```python
from build123d import *

# Parameters (mm, degrees)
SKETCH1_R           = 381
BOSS_EXTRUDE1_DEPTH = 12.7
SKETCH6_R           = 15.25
CUT_EXTRUDE1_DEPTH  = 12.7


with BuildPart() as part:
    # Sketch1 → Boss-Extrude1 (new body, symmetric)
    with BuildSketch(Plane(origin=(0, 0, 0), x_dir=(1, 0, 0), z_dir=(0, 1, 0))):
        Circle(SKETCH1_R)
    extrude(amount=BOSS_EXTRUDE1_DEPTH, both=True)

    # Sketch6 → Cut-Extrude1 (cut)
    with BuildSketch(Plane(origin=(0, 12.7, 0), x_dir=(1, 0, 0), z_dir=(0, 1, 0))):
        Circle(SKETCH6_R)
        with Locations((-101.6, 0)):
            Circle(SKETCH6_R)
        with Locations((101.6, 0)):
            Circle(SKETCH6_R)
        with Locations((-101.6, 101.6)):
            Circle(SKETCH6_R)
        with Locations((0, 101.6)):
            Circle(SKETCH6_R)
        with Locations((101.6, 101.6)):
            Circle(SKETCH6_R)
        with Locations((-101.6, -101.6)):
            Circle(SKETCH6_R)
        with Locations((0, -101.6)):
            Circle(SKETCH6_R)
        with Locations((101.6, -101.6)):
            Circle(SKETCH6_R)
        with Locations((101.6, 203.2)):
            Circle(SKETCH6_R)
        with Locations((0, 203.2)):
            Circle(SKETCH6_R)
        with Locations((-101.6, 203.2)):
            Circle(SKETCH6_R)
        with Locations((101.6, 304.8)):
            Circle(SKETCH6_R)
        with Locations((0, 304.8)):
            Circle(SKETCH6_R)
        with Locations((-101.6, 304.8)):
            Circle(SKETCH6_R)
        with Locations((101.6, -203.2)):
            Circle(SKETCH6_R)
        with Locations((0, -203.2)):
            Circle(SKETCH6_R)
        with Locations((-101.6, -203.2)):
            Circle(SKETCH6_R)
        with Locations((101.6, -304.8)):
            Circle(SKETCH6_R)
        with Locations((0, -304.8)):
            Circle(SKETCH6_R)
        with Locations((-101.6, -304.8)):
            Circle(SKETCH6_R)
        with Locations((203.2, -101.6)):
            Circle(SKETCH6_R)
        with Locations((203.2, 0)):
            Circle(SKETCH6_R)
        with Locations((203.2, 101.6)):
            Circle(SKETCH6_R)
        with Locations((304.8, -101.6)):
            Circle(SKETCH6_R)
        with Locations((304.8, 0)):
            Circle(SKETCH6_R)
        with Locations((304.8, 101.6)):
            Circle(SKETCH6_R)
        with Locations((-203.2, 101.6)):
            Circle(SKETCH6_R)
        with Locations((-203.2, 0)):
            Circle(SKETCH6_R)
        with Locations((-203.2, -101.6)):
            Circle(SKETCH6_R)
        with Locations((-304.8, 101.6)):
            Circle(SKETCH6_R)
        with Locations((-304.8, 0)):
            Circle(SKETCH6_R)
        with Locations((-304.8, -101.6)):
            Circle(SKETCH6_R)
        with Locations((-203.2, 203.2)):
            Circle(SKETCH6_R)
        with Locations((203.2, 203.2)):
            Circle(SKETCH6_R)
        with Locations((203.2, -203.2)):
            Circle(SKETCH6_R)
        with Locations((-203.2, -203.2)):
            Circle(SKETCH6_R)
    extrude(amount=-CUT_EXTRUDE1_DEPTH, mode=Mode.SUBTRACT)


solid = part.part
```
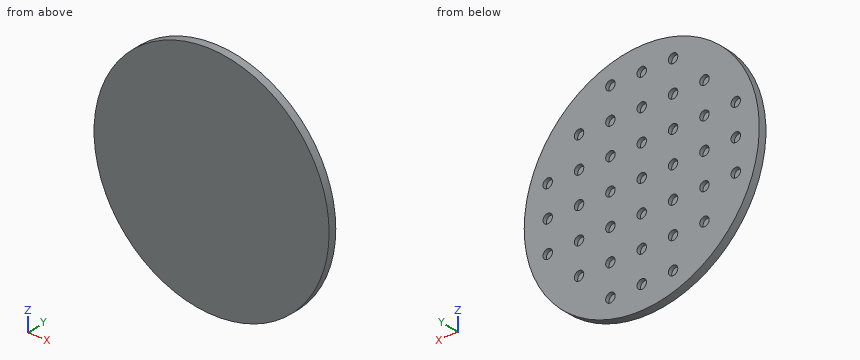
Design review of the part built by this model. Coordinates are the model's own, in mm. Give positions to 0.01 mm unless a question says otherwise; leave off trailing zeros. Loops run counter-clockwise (first coordinate to the right, second up) from the corner with the lowest first, then second, coordinate; pieces in that order, holes last. Notation, with made-up numbers: M 31.25,63.5 L 65.25,63.5 A9 cw 65.25,79.5 Z; hole C 11,37.5 d7. An arc over 180 degrees is marked long. Return JSON: item names as keys, results as strings. Group by question number.
Item 1: Insertion check: pin 1 Ø9 at (x, z) = (-201.5, 4) entering from +Y; pin 2 Ø5 at (y, z) = (-2, -121.5) entering from +X; pin 3 Ø6 at (x, y) = (-231, 5) entering from +Z. Each pin has a flat end and moves straight along its axis. Give the tip position at first contact, or say it passes through.
Item 2: We need section B-B (x = -304.8). Give the boundary of the cut face in (y, z).
Item 3: We need section A-A (z = -304.8). Give the boundary of the cut face in (x, y).
Item 4: We need section C-C (y = -6.25). Give the boundary of the cut face in (x, z), and give its area (3 significant figures).
Item 5: For probe 1 along X at (y, z) = (8.5, -312); probe 2 along X at (y, z) = (3.75, 203.2); probe 3 along X at (y, z) = (5.5, -192), list the stretches that pass through material, from the lowest coordinate up.
Output:
{
 "1": {"pin 1": "stops at y = 0", "pin 2": "stops at x = 361.94", "pin 3": "stops at z = 305.25"},
 "2": {"outline": "M -12.7,-228.6 L 12.7,-228.6 L 12.7,-116.85 L 0,-116.85 L 0,-86.35 L 12.7,-86.35 L 12.7,-15.25 L 0,-15.25 L 0,15.25 L 12.7,15.25 L 12.7,86.35 L 0,86.35 L 0,116.85 L 12.7,116.85 L 12.7,228.6 L -12.7,228.6 Z"},
 "3": {"outline": "M -228.6,-12.7 L 228.6,-12.7 L 228.6,12.7 L 116.85,12.7 L 116.85,0 L 86.35,0 L 86.35,12.7 L 15.25,12.7 L 15.25,0 L -15.25,0 L -15.25,12.7 L -86.35,12.7 L -86.35,0 L -116.85,0 L -116.85,12.7 L -228.6,12.7 Z"},
 "4": {"outline": "C 0,0 d762", "area": "456,000 mm^2"},
 "5": {"probe 1": "x = -218.67 to -115.04, -88.16 to -13.44, 13.44 to 88.16, 115.04 to 218.67", "probe 2": "x = -322.29 to -218.45, -187.95 to -116.85, -86.35 to -15.25, 15.25 to 86.35, 116.85 to 187.95, 218.45 to 322.29", "probe 3": "x = -329.09 to -213.55, -192.85 to -111.95, -91.25 to -10.35, 10.35 to 91.25, 111.95 to 192.85, 213.55 to 329.09"}
}
